Verification items for the finished model (mm, model axes). A direction names the side the tool comes from. Round coordinates to 2 decimals unless told otherwise and drop trailing zeros. Loops run counter-clockwise (first coordinate to the right, second up) from the corner with the lowest first, then second, coordinate; pieces in that order, holes last. Notation, with made-up numbers: (-10, 26) - (13, 26) arc R33 cw to (13, 63) - close; hole circle Ø11 at (-37, -17.5). An arc over 180 degrees is marked (long way). Use CSV: the item, a comma, the result in double quotes.
```python
from build123d import *

# Parameters (mm, degrees)
SKETCH1_R           = 5.35
BOSS_EXTRUDE2_DEPTH = 7
SKETCH8_R           = 2.375
CUT_EXTRUDE2_DEPTH  = 2.25
BOSS_EXTRUDE3_DEPTH = 22
SKETCH10_W          = 82.482524805
SKETCH10_H          = 7
BOSS_EXTRUDE4_DEPTH = 5
CHAMFER1_SIZE       = 5
SKETCH11_W          = 39.19
SKETCH11_H          = 3
SKETCH11_W_2        = 21.55
CUT_EXTRUDE3_DEPTH  = 15
SKETCH12_W          = 23.17
SKETCH12_H          = 7.7
SKETCH12_H_2        = 3.2
BOSS_EXTRUDE5_DEPTH = 7


with BuildPart() as part:
    # Sketch1 → Boss-Extrude2 (new body)
    with BuildSketch(Plane.XY):
        Polygon((-19.503784034, -20), (19.503784034, -20), (62.978740771, -20), (62.978740771, 13), (19.503784034, 13), (-19.503784034, 13), align=None)
        Circle(SKETCH1_R, mode=Mode.SUBTRACT)
    extrude(amount=-BOSS_EXTRUDE2_DEPTH)

    # Sketch8 → Cut-Extrude2 (cut)
    with BuildSketch(Plane(origin=(0, 0, -7), x_dir=(-1, 0, 0), z_dir=(0, 0, -1))):
        with Locations((-11.35, 0)):
            Circle(SKETCH8_R)
    extrude(amount=-CUT_EXTRUDE2_DEPTH, mode=Mode.SUBTRACT)

    # Sketch9 → Boss-Extrude3 (add)
    with BuildSketch(Plane(origin=(0, 0, -7), x_dir=(-1, 0, 0), z_dir=(0, 0, -1))):
        Polygon((12.003784034, 3.25), (12.003784034, 13), (19.503784034, 13), (19.503784034, -12.662545792), (19.503784034, -20), (-56.5, -20), (-62.978740771, -20), (-62.978740771, 13), (-51.996215966, 13), (-51.996215966, 5), (-53.996215966, 5), (-53.996215966, -5), (-51.996215966, -5), (-51.996215966, -11.25), (12.003784034, -11.25), (12.003784034, -3.25), (17.003784034, -3.25), (17.003784034, 3.25), align=None)
    extrude(amount=BOSS_EXTRUDE3_DEPTH)

    # Sketch10 → Boss-Extrude4 (add)
    with BuildSketch(Plane(origin=(0, 13, 0), x_dir=(1, 0, 0), z_dir=(0, 1, 0))):
        with Locations((21.737478368, 3.5)):
            Rectangle(SKETCH10_W, SKETCH10_H)
    extrude(amount=BOSS_EXTRUDE4_DEPTH)

    # Chamfer1
    chamfer1_edges = [part.edges().sort_by_distance(p)[0] for p in [
        (62.978740771, 18, -3.5),
        (-19.503784034, 18, -3.5),
    ]]
    chamfer(chamfer1_edges, length=CHAMFER1_SIZE)

    # Sketch11 → Cut-Extrude3 (cut)
    with BuildSketch(Plane(origin=(0, 0, -29), x_dir=(-1, 0, 0), z_dir=(0, 0, -1))):
        Polygon((-60.239370385, 10), (-58.487478368, 10), (-58.487478368, 13), (-56.487478368, 13), (-56.487478368, 10), (-54.239370385, 10), (-54.239370385, 8), (-60.239370385, 8), align=None)
        with Locations((-40.644370385, -15.5)):
            Rectangle(SKETCH11_W, SKETCH11_H)
        with Locations((5.978784034, -15.5)):
            Rectangle(SKETCH11_W_2, SKETCH11_H)
        Polygon((14.753784034, 13), (16.753784034, 13), (16.753784034, 10), (18.753784034, 10), (18.753784034, 8), (12.753784034, 8), (12.753784034, 10), (14.753784034, 10), align=None)
    extrude(amount=-CUT_EXTRUDE3_DEPTH, mode=Mode.SUBTRACT)

    # Sketch12 → Boss-Extrude5 (add)
    with BuildSketch(Plane.XY):
        with Locations((36.243740771, -7.15)):
            Rectangle(SKETCH12_W, SKETCH12_H)
        with Locations((36.243740771, 3.6)):
            Rectangle(SKETCH12_W, SKETCH12_H_2)
    extrude(amount=BOSS_EXTRUDE5_DEPTH)


solid = part.part
```
1) Thickness scan on probe 1 along X at (y, z) = (-15.5, -16.5); probe 2 along Y at (x, z) = (-13.5, -15.5); probe 3 along Y at (x, z) = (0, -5). Record the ranges inside material, lowest first. Write a range as [from, to].
Returned:
probe 1,"x = [-19.5, -16.75], [4.8, 21.05], [60.24, 62.98]"
probe 2,"y = [-20, -17], [-14, -3.25], [3.25, 8], [10, 13]"
probe 3,"y = [-20, -5.35], [5.35, 18]"
2) Cross-section at C-C, the plane y = 0. Record the cut outline in (x, z) (3 decimals).
Returned:
outline,"(-19.504, -29) - (-17.004, -29) - (-17.004, -7) - (-5.35, -7) - (-5.35, 0) - (-19.504, 0) - close; (5.35, -7) - (8.975, -7) - (8.975, -4.75) - (13.725, -4.75) - (13.725, -7) - (53.996, -7) - (53.996, -29) - (62.979, -29) - (62.979, 0) - (5.35, 0) - close"
3) Cross-section at B-B, the plane x = 0. Record the cut outline in (y, z).
Returned:
outline,"(-20, -29) - (-17, -29) - (-17, -14) - (-14, -14) - (-14, -29) - (-11.25, -29) - (-11.25, -7) - (-5.35, -7) - (-5.35, 0) - (-20, 0) - close; (5.35, -7) - (18, -7) - (18, 0) - (5.35, 0) - close"
4) Cross-section at D-D, the plane x = 28. Record the cut outline in (y, z), then the cut area to 3 significant figures.
Returned:
outline,"(-20, -29) - (-17, -29) - (-17, -14) - (-14, -14) - (-14, -29) - (-11.25, -29) - (-11.25, -7) - (18, -7) - (18, 0) - (5.2, 0) - (5.2, 7) - (2, 7) - (2, 0) - (-3.3, 0) - (-3.3, 7) - (-11, 7) - (-11, 0) - (-20, 0) - close"
area,"490 mm²"
5) Access from +Z, -Z, +X, -X, +Y, -Y to the whole of each face (thin tool, end or side, straight path). Record for faces 5 (the face through (-1.16, -5.223, -3.451)), 6 (the face through (-14, -3.25, -18)).
Returned:
face 5,"+Z, -Z"
face 6,"-Z"
6) Mould release check, pull along Y, two halves, no side actions. Record for faces 1 (the face through (22, -20, -14)), 2 (the face through (62.979, -4, -14)), 3 (the face through (20, -11.25, -18)), 4 (the face through (-6, -15, -14)): +Y half, -Y half, draft (parallel to the pull), parting line (faces both ways), or undercut.
Returned:
face 1,"-Y half"
face 2,"draft"
face 3,"+Y half"
face 4,"undercut"
7) Cross-section at A-A, the plane z = 5. Record the cut outline in (x, y), then the cut area to 3 significant figures.
Returned:
outline,"(24.66, -11) - (47.83, -11) - (47.83, -3.3) - (24.66, -3.3) - close; (24.66, 2) - (47.83, 2) - (47.83, 5.2) - (24.66, 5.2) - close"
area,"253 mm²"
8) Gauge pin test, flat ends, axial feed: pin 1 Ø12.5 at (x, y) = (0, 0) entering from -Z; pin 2 Ø1.8 at (x, z) = (58.5, -24.5) entering from +Y; pin 3 Ø5 at (x, y) = (3, -3) entering from +Z. Record the tip position at first contact, or that the pin passes through.
Returned:
pin 1,"stops at z = -7"
pin 2,"stops at y = 13"
pin 3,"stops at z = 0"
